For this review, use the dimensioned drawing (mm, ordinates from the lowest corner) and the shaded views. A direction names the side the tool comes from. Give positions to 0.01 mm unless a question says otherwise; leave off trailing zeros. Write each loop counter-clockwise with the first axis right and the second up, starting at its lowest first coordinate (ties: lowest second). Pieces come first, ordered by that corner, then holes. Notation, with made-up numbers: (4.5, 86) -> (59.5, 86) arc R19 cw to (59.5, 107) -> close; hole circle Ø2 at (33, 27.25). An arc over 180 degrees is marked (long way). Write each question's results on one line, items separated by ' | '. Start each with the question number.
(1) Take a section at C-C (y = 30). State the section outline as (x, z) points.
(2) Take a section at D-D (x = 43). State the section outline as (y, z) points, plus the area to 3 significant figures.
(3) To check wall thickness, follow probe 1 along Y at (x, z) = (41.5, 11.5); probe 2 along X at (y, z) = (40, 23); probe 3 along Z at (x, y) = (23.5, 43). State the ranges of each line that lie inside material, in increasing order.
(4) For the marked faces 1 and 2, list the 3-axis set-ups (+Z, -Z, +X, -X, +Y, -Y) from which the entire face can be reached by the end or side of a thin tool; tool diameter is ignored.
(5) Take a section at A-A (x = 25). State the section outline as (y, z) points, plus the area to 3 significant figures.
(6) Take a section at B-B (z = 25). State the section outline as (x, y) points.
(7) Clearance check with flat-ended pins moving along their axes: pin 1 (4 mm diameter, centred on x = 19.5, z = 31, fed in from -Y); pin 2 (5 mm diameter, centred on x = 17.5, y = 19.5, fed in from +Z); pin 3 (2 mm diameter, centred on x = 25, z = 35.5, fed in from +Y); pin 4 (12 mm diameter, centred on x = 22.5, y = 37.5, fed in from -Z). State where each tip first meets the part, or that it passes through.
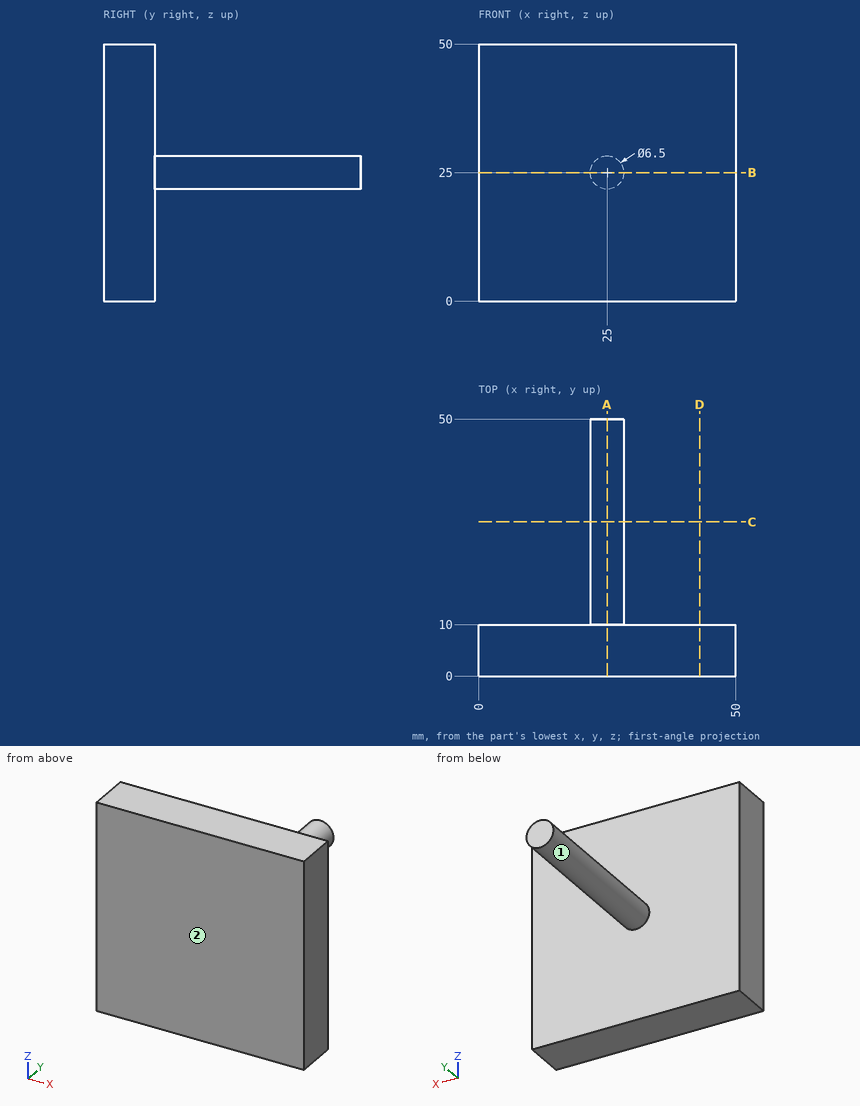
Report:
1) outline: circle Ø6.5 at (25, 25)
2) outline: (0, 0) -> (10, 0) -> (10, 50) -> (0, 50) -> close | area: 500 mm2
3) probe 1: 0 to 10 | probe 2: 22.44 to 27.56 | probe 3: 22.12 to 27.88
4) face 1: +Y | face 2: +Z, -Z, +X, -X, -Y
5) outline: (0, 0) -> (10, 0) -> (10, 21.75) -> (50, 21.75) -> (50, 28.25) -> (10, 28.25) -> (10, 50) -> (0, 50) -> close | area: 760 mm2
6) outline: (0, 0) -> (50, 0) -> (50, 10) -> (28.25, 10) -> (28.25, 50) -> (21.75, 50) -> (21.75, 10) -> (0, 10) -> close
7) pin 1: y = 0 | pin 2: through | pin 3: y = 10 | pin 4: z = 21.75
